Build history of the part. All positions in model axes, mm. Face numbers are marked on the shaded views. Coordinates: 2 decimals unless noted, no trailing zeros. Loops run counter-clockwise (first coordinate to the right, second up) from the corner with the lowest first, then second, coordinate; pieces in that order, holes last.
Item 1: Cut at B-B (z = 0.75). List the corners of the cut face in (x, y) (3 decimals), and give its area (3 significant figures).
Item 2: Drill centre lines: line 1 along X through (y, z) = (60, 3.6); line 2 along Y through (x, z) = (13, 1.5); line 3 along Y through (x, z) = (14, 2.1). Where is each one in solid material? Low to high.
Item 3: Cut at D-D (x = -15). List the corners of the cut face in (y, z), and give its area (3 significant figures).
Item 4: Flat gauge pins, fed straight in: pin 1 (4 mm diameter, centred on x = 4, y = 78.5, fed in from -Z); pin 2 (5 mm diameter, centred on x = 11.54, y = 5.1, fed in from +Z); pin 3 (3 mm diameter, centred on y = 99.5, z = 1.5, fed in from -X); pin 4 (3 mm diameter, centred on x = -19, z = 2.5, fed in from +Y). Where does each tip first touch, or does it go through?
Item 5: Cut at C-C (y = 18.5). List the corners of the cut face in (x, z).
Item 6: Mould opens along X. For the marked faces 1 and 2 say: released by +X, released by -X, zero draft, split by the parting line, or undercut.
Item 7: Cut at A-A (x = 12.5). List the corners of the cut face in (y, z).
from build123d import *

# Parameters (mm, degrees)
EXTRUDE_1_DEPTH     = 5
SKETCH_2_R          = 4
CUT_EXTRUDE_1_DEPTH = 5
SKETCH_3_R          = 4
EXTRUDE_2_DEPTH     = 5


with BuildPart() as part:
    # 草图1 → 凸台-拉伸1 (new body)
    with BuildSketch(Plane.XY):
        Polygon((0, 0), (0, 65), (-48.75546427, 110.693878657), (23.07, 65), (23.07, 0), align=None)
    extrude(amount=EXTRUDE_1_DEPTH)

    # 草图2 → 切除-拉伸1 (cut)
    with BuildSketch(Plane.XY.offset(5)):
        with Locations((11.535, 5.104320519)):
            Circle(SKETCH_2_R)
        with Locations(Location((11.535, 59.895679481, 0), (0, 0, 180))):
            Circle(SKETCH_2_R)
    extrude(amount=-CUT_EXTRUDE_1_DEPTH, mode=Mode.SUBTRACT)

    # 草图3 → 凸台-拉伸2 (add)
    with BuildSketch(Plane.XY.offset(5)):
        with Locations((11.535, 59.895679481)):
            Circle(SKETCH_3_R)
    extrude(amount=-EXTRUDE_2_DEPTH)


solid = part.part
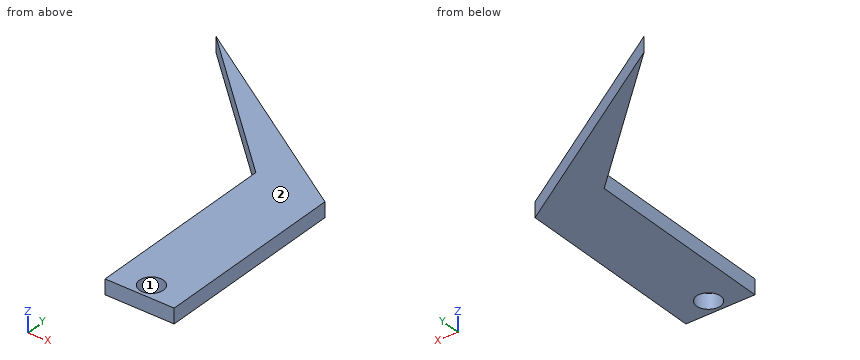
Filled sheet:
1. outline: (-48.755, 110.694) - (0, 65) - (0, 0) - (23.07, 0) - (23.07, 65) - close; hole circle Ø8 at (11.535, 5.104)
1. area: 1,980 mm2
2. line 1: x = 0 to 23.07
2. line 2: y = 0 to 1.38, 8.83 to 71.41
2. line 3: y = 0 to 1.95, 8.25 to 70.77
3. outline: (79.06, 0) - (89.22, 0) - (89.22, 5) - (79.06, 5) - close
3. area: 50.8 mm2
4. pin 1: stops at z = 0
4. pin 2: passes through
4. pin 3: stops at x = -38.41
4. pin 4: stops at y = 92.72
5. outline: (0, 0) - (23.07, 0) - (23.07, 5) - (0, 5) - close
6. face 1: undercut
6. face 2: zero draft
7. outline: (0, 0) - (1.22, 0) - (1.22, 5) - (0, 5) - close; (8.99, 0) - (71.72, 0) - (71.72, 5) - (8.99, 5) - close
